Geometry: see drawing. Coordinates: mm, zero at the bounding-box minimum. Give positions to 0.01 mm unless a question says otherwise; leave off trailing zeros. Loops run counter-clockwise (first coordinate to the right, second up) from the corner with the lowest first, then second, coordinate; pieces in that order, holes last. Notation, with made-up numbers: M -9.75,-13.5 L 45.25,-13.5 A24 cw 45.25,15.5 Z; hole C 50,74 d2. An arc over 180 degrees is marked long. Answer in a Markdown table with one row per item.
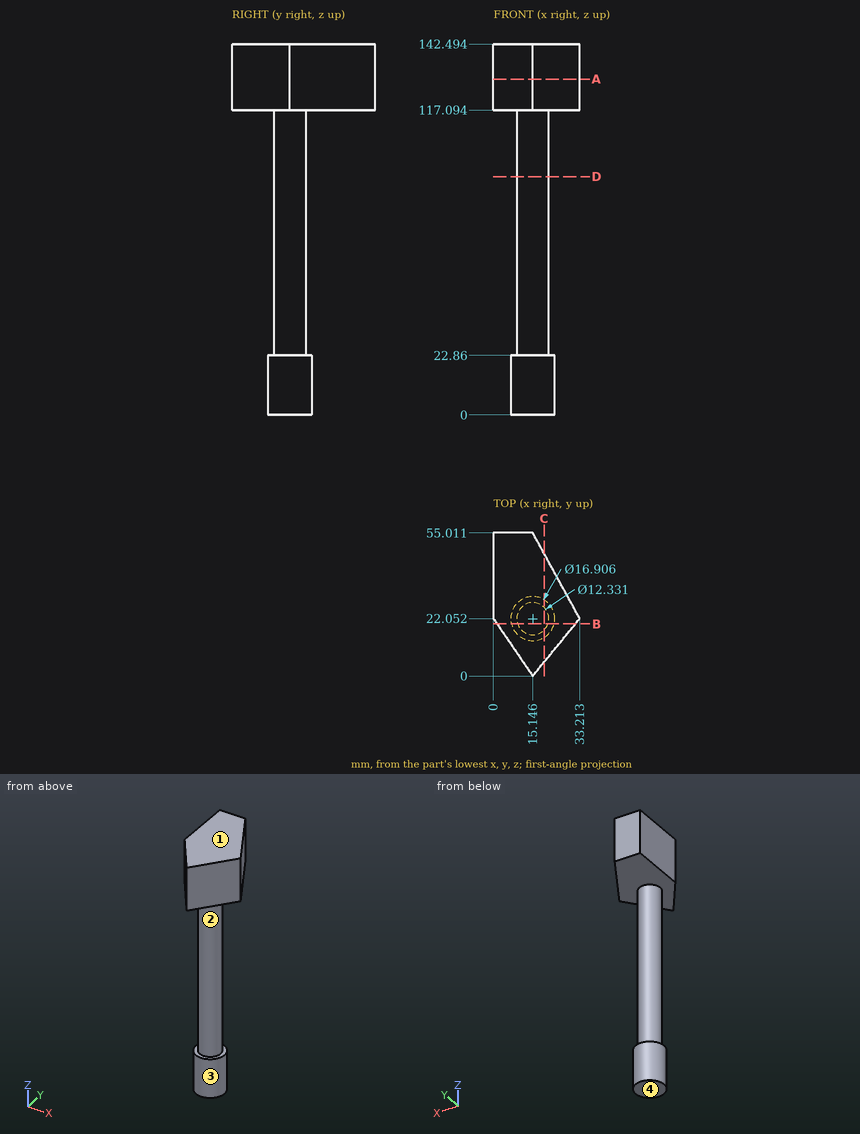
1) Section D-D, the plane z = 91.5. Return loops of the section in (x, y) (1 decimal), then the cut area to 3 significant figures.
Reply:
| item | result |
|---|---|
| outline | C 15.1,22.1 d12.3 |
| area | 119 mm² |
2) Section B-B, the plane y = 20. Return loops of the section in (x, z) (1 decimal).
Reply:
| item | result |
|---|---|
| outline | M 1.4,117.1 L 9.3,117.1 L 9.3,22.9 L 6.9,22.9 L 6.9,0 L 23.3,0 L 23.3,22.9 L 21,22.9 L 21,117.1 L 31.5,117.1 L 31.5,142.5 L 1.4,142.5 Z |
3) Section A-A, the plane z = 129. Return loops of the section in (x, y), then the cut area to 3 significant figures.
Reply:
| item | result |
|---|---|
| outline | M 0,22.05 L 15.15,0 L 33.21,22.05 L 15.15,55.01 L 0,55.01 Z |
| area | 1,160 mm² |
4) Pull-direction query (Z, two-part tool) for the marked faces 1, 2, 3 and 4; classes: released by +Z, released by -Z, zero draft, split by the parting line, or undercut.
Reply:
| item | result |
|---|---|
| face 1 | released by +Z |
| face 2 | undercut |
| face 3 | zero draft |
| face 4 | released by -Z |
5) Section C-C, the plane x = 19.5. Return loops of the section in (y, z) (1 decimal).
Reply:
| item | result |
|---|---|
| outline | M 5.3,117.1 L 17.7,117.1 L 17.7,22.9 L 14.8,22.9 L 14.8,0 L 29.3,0 L 29.3,22.9 L 26.4,22.9 L 26.4,117.1 L 47.1,117.1 L 47.1,142.5 L 5.3,142.5 Z |
6) Pin query (flat end, axial travel): pin 1 Ø6 at (x, y) = (15, 35.5) entering from -Z; pin 2 Ø4 at (x, z) = (16.5, 16) entering from -Y; pin 3 Ø10 at (x, y) = (8.5, 19) entering from -Z; pin 4 Ø10 at (x, z) = (6.5, 105) entering from +Y (1 decimal). Return the tip coordinate at first contact, or that it passes through.
Reply:
| item | result |
|---|---|
| pin 1 | stops at z = 117.09 |
| pin 2 | stops at y = 13.6 |
| pin 3 | stops at z = 0 |
| pin 4 | stops at y = 27 |
7) Material intervals for L1, parallel to Z at x = 9, y = 31 (1 decimal); L2, parallel to Y at x = 19, z = 7.5 (1 decimal); L3, parallel to X at y = 17.5, z = 123.5 (1 decimal), sorted ascending.
Reply:
| item | result |
|---|---|
| L1 | z = 117.1 to 142.5 |
| L2 | y = 14.5 to 29.6 |
| L3 | x = 3.1 to 29.5 |
